from build123d import *

# Parameters (mm, degrees)
SKETCH1_R           = 2.75
BOSS_EXTRUDE1_DEPTH = 7.5
BOSS_EXTRUDE2_DEPTH = 98
FILLET1_R           = 3
SKETCH4_R           = 25
BOSS_EXTRUDE4_DEPTH = 3
SKETCH5_R           = 7
BOSS_EXTRUDE5_DEPTH = 27


with BuildPart() as part:
    # Sketch1 → Boss-Extrude1 (new body)
    with BuildSketch(Plane(origin=(0, 0, 0), x_dir=(1, 0, 0), z_dir=(0, 1, 0))):
        with BuildLine():
            Line((-27, -30), (27, -30))
            ThreePointArc((27, -30), (29.121320344, -29.121320344), (30, -27))
            Line((30, -27), (30, 27))
            ThreePointArc((30, 27), (29.121320344, 29.121320344), (27, 30))
            Line((27, 30), (-27, 30))
            ThreePointArc((-27, 30), (-29.121320344, 29.121320344), (-30, 27))
            Line((-30, 27), (-30, -27))
            ThreePointArc((-30, -27), (-29.121320344, -29.121320344), (-27, -30))
        make_face()
        with Locations(Location((-24.748737342, 24.748737342, 0), (0, 0, 270))):
            Circle(SKETCH1_R, mode=Mode.SUBTRACT)
        with Locations(Location((24.748737342, 24.748737342, 0), (0, 0, 270))):
            Circle(SKETCH1_R, mode=Mode.SUBTRACT)
        with Locations(Location((-24.748737342, -24.748737342, 0), (0, 0, 90))):
            Circle(SKETCH1_R, mode=Mode.SUBTRACT)
        with Locations(Location((24.748737342, -24.748737342, 0), (0, 0, 90))):
            Circle(SKETCH1_R, mode=Mode.SUBTRACT)
    extrude(amount=BOSS_EXTRUDE1_DEPTH)

    # Sketch2 → Boss-Extrude2 (add)
    with BuildSketch(Plane(origin=(0, 7.5, 0), x_dir=(1, 0, 0), z_dir=(0, 1, 0))):
        Polygon((-20, 30), (20, 30), (20, 20), (30, 20), (30, -20), (20, -20), (20, -30), (-20, -30), (-20, -20), (-30, -20), (-30, 20), (-20, 20), align=None)
    extrude(amount=BOSS_EXTRUDE2_DEPTH)

    # Fillet1
    fillet1_edges = [part.edges().sort_by_distance(p)[0] for p in [
        (-20, 56.5, -30),
        (-20, 56.5, -20),
        (-30, 56.5, -20),
        (-30, 56.5, 20),
        (-20, 56.5, 20),
        (-20, 56.5, 30),
        (20, 56.5, 30),
        (20, 56.5, 20),
        (30, 56.5, 20),
        (30, 56.5, -20),
        (20, 56.5, -20),
        (20, 56.5, -30),
    ]]
    fillet(fillet1_edges, radius=FILLET1_R)

    # Sketch4 → Boss-Extrude4 (add)
    with BuildSketch(Plane.XZ):
        with Locations(Location((0, 0, 0), (0, 0, 270))):
            Circle(SKETCH4_R)
    extrude(amount=BOSS_EXTRUDE4_DEPTH)

    # Sketch5 → Boss-Extrude5 (add)
    with BuildSketch(Plane.XZ.offset(3)):
        with Locations(Location((0, 0, 0), (0, 0, 270))):
            Circle(SKETCH5_R)
    extrude(amount=BOSS_EXTRUDE5_DEPTH)


solid = part.part
Could you check a few things on this model? Use its own coordinates, in mm. A direction names the side the tool comes from. Give positions to 0.01 mm unless a question says otherwise; leave off trailing zeros. Order: outer loops, then holes, each group sorted by start corner. A loop starts at its lowest first (then second) coordinate and runs counter-clockwise, first axis right, second up. Notation, with made-up numbers: (51.25, 36) - (59.25, 36) arc R26 ccw to (59.25, 50) - close; hole circle Ø1 at (49.25, 50). An arc over 180 degrees is marked (long way). Return JSON: item names as keys, results as strings. Group by question number.
Q1. Which directions (+Z, -Z, +X, -X, +Y, -Y) give clear straight access to the entire face, cutting with the end or side of a thin tool? Please do faces 1 (the face through (29.14, 57.19, -19.1)), 2 (the face through (20, 56, 25)), 3 (the face through (-20, 56, 25)).
Q2. Thinking about a two-plate mould opening in X: for faces 4 (the face through (-22.064, 3.698, 25.345)), 5 (the face through (19.1, 57.19, -29.14)), 6 (the face through (-20, 56, -25)), which applies, pulls with the +X half, pulls with the -X half, needs draft (parallel to the pull), parting line crosses it, or undercut?
Q3. Suppose I cut it at D-D, the plane x = 9. Please give me the cut outline in (y, z), and give its area (3 significant figures).
Q4. Please list where these lines run through material, in increasing order: line 1 along Z through (x, y) = (23.5, 7); line 2 along Y through (x, z) = (-10, 26); line 3 along Y through (x, z) = (20, 2). Write a range as [from, to].
Q5. Suppose I cut it at A-A, the plane y = 56.5. Please give me the cut outline in (x, z), and give its area (3 significant figures).
Q6. Suppose I cut it at C-C, the plane z = 0. Please give me the cut outline in (x, y).
Q7. Suppose I cut it at B-B, the plane x = 0. Please give me the cut outline in (y, z), and give its area (3 significant figures).
Q8. Will these pins go through, and if not, where does the flat tip stop? pin 1 Ø4.5 at (x, y) = (-26, 38.5) entering from +Z; pin 2 Ø1.2 at (y, z) = (40.5, -24.5) entering from -X; pin 3 Ø3 at (y, z) = (76, -24.5) entering from +X; pin 4 Ø12 at (x, z) = (-1.5, 10) entering from -Y.
Resolved:
{
 "1": {"face 1": "-Z, +X, +Y", "face 2": "+Z, +X, +Y", "face 3": "+Z, -X, +Y"},
 "2": {"face 4": "undercut", "face 5": "pulls with the +X half", "face 6": "pulls with the -X half"},
 "3": {"outline": "(-3, -23.32) - (0, -23.32) - (0, -30) - (105.5, -30) - (105.5, 30) - (0, 30) - (0, 23.32) - (-3, 23.32) - close", "area": "6,470 mm2"},
 "4": {"line 1": "z = [-30, -27.2], [-22.3, 22.3], [27.2, 30]", "line 2": "y = [0, 105.5]", "line 3": "y = [-3, 105.5]"},
 "5": {"outline": "(-30, -17) arc R3 ccw to (-27, -20) - (-23, -20) arc R3 cw to (-20, -23) - (-20, -27) arc R3 ccw to (-17, -30) - (17, -30) arc R3 ccw to (20, -27) - (20, -23) arc R3 cw to (23, -20) - (27, -20) arc R3 ccw to (30, -17) - (30, 17) arc R3 ccw to (27, 20) - (23, 20) arc R3 cw to (20, 23) - (20, 27) arc R3 ccw to (17, 30) - (-17, 30) arc R3 ccw to (-20, 27) - (-20, 23) arc R3 cw to (-23, 20) - (-27, 20) arc R3 ccw to (-30, 17) - close", "area": "3,190 mm2"},
 "6": {"outline": "(-30, 0) - (-25, 0) - (-25, -3) - (-7, -3) - (-7, -30) - (7, -30) - (7, -3) - (25, -3) - (25, 0) - (30, 0) - (30, 105.5) - (-30, 105.5) - close"},
 "7": {"outline": "(-30, -7) - (-3, -7) - (-3, -25) - (0, -25) - (0, -30) - (105.5, -30) - (105.5, 30) - (0, 30) - (0, 25) - (-3, 25) - (-3, 7) - (-30, 7) - close", "area": "6,860 mm2"},
 "8": {"pin 1": "stops at z = 20", "pin 2": "stops at x = -20", "pin 3": "stops at x = 20", "pin 4": "stops at y = -30"}
}
